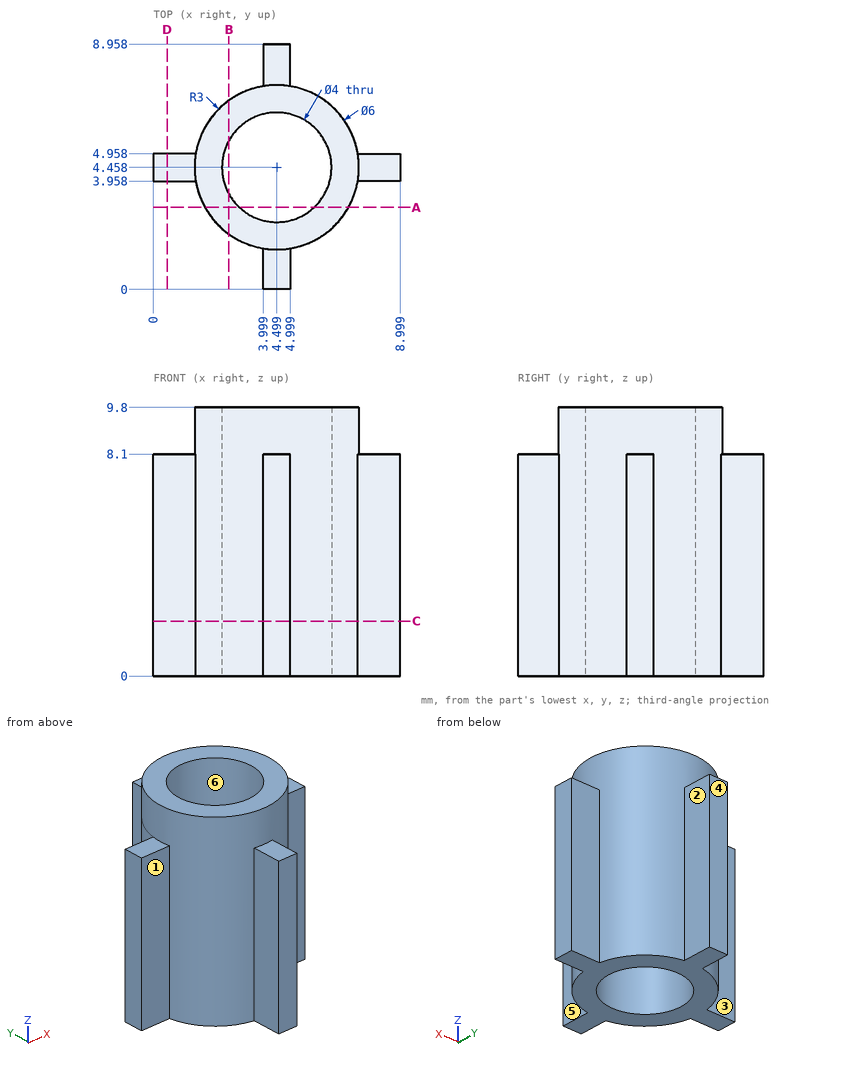
Can you work these out from the drawing? Everything is in mm from the part's minimum corner. A direction names the side the tool comes from. Give positions to 0.01 mm unless a question says otherwise; leave off trailing zeros. Write each loop counter-clockwise with the first axis right and the second up, starting at its lowest first coordinate (ties: lowest second). Pieces come first, ordered by that corner, then holes. Notation, with made-up numbers: (-3, -39.75) -> (24, -39.75) arc R12 ccw to (24, -16.75) -> close; hole circle Ø9 at (52.5, -4). An arc over 180 degrees is marked (long way). Write each question's results on one line, items separated by ' | '. Start each with the question number.
Q1. We'd pull the mould along Y, two halves only. Please class the marked faces 4, 5 and 6: +Y half, -Y half, draft (parallel to the pull), parting line (faces both ways), or undercut.
Q2. Suppose I cut it at A-A, the plane y = 3. List the corners of the cut face in (x, z) for me.
Q3. I'm going to push flat-ended pins straight in: pin 1 Ø0.5 at (x, z) = (8, 4) entering from -Y; pin 2 Ø0.8 at (y, z) = (0.5, 6) entering from +X; pin 3 Ø0.8 at (x, z) = (8.5, 5) entering from +Y. Where does each tip first touch, or does it pass through?
Q4. Suppose I cut it at B-B, the plane x = 2.75. List the corners of the cut face in (y, z) for me.
Q5. I need wall thicknesses on probe 1 along Y at (x, z) = (4.5, 9); probe 2 along X at (y, z) = (4.5, 7); probe 3 along X at (y, z) = (3.5, 9.75) (1 decimal). Which ranges of each line are inside material? Lowest first, please.
Q6. Which directions (+Z, -Z, +X, -X, +Y, -Y) give clear straight access to the entire face, cutting with the end or side of a thin tool? Please do the marked faces 1, 2 and 3.
Q7. Suppose I cut it at D-D, the plane x = 0.5. List the corners of the cut face in (y, z) for me.
Q8. Suppose I cut it at C-C, the plane z = 2. List the corners of the cut face in (x, y) for me, and give its area (3 significant figures).
Outcome:
1) face 4: +Y half | face 5: draft | face 6: undercut
2) outline: (1.88, 0) -> (3.13, 0) -> (3.13, 9.8) -> (1.88, 9.8) -> close; (5.87, 0) -> (7.12, 0) -> (7.12, 9.8) -> (5.87, 9.8) -> close
3) pin 1: y = 3.96 | pin 2: x = 5 | pin 3: y = 4.96
4) outline: (2.02, 0) -> (3.49, 0) -> (3.49, 9.8) -> (2.02, 9.8) -> close; (5.43, 0) -> (6.9, 0) -> (6.9, 9.8) -> (5.43, 9.8) -> close
5) probe 1: 1.46 to 2.46, 6.46 to 7.46 | probe 2: 0 to 2.5, 6.5 to 9 | probe 3: 1.7 to 2.7, 6.3 to 7.3
6) face 1: +Z, -Z, -X, -Y | face 2: +Z, -Z, +X, +Y | face 3: +Z, -Z, -X, +Y
7) outline: (3.96, 0) -> (4.96, 0) -> (4.96, 8.1) -> (3.96, 8.1) -> close
8) outline: (0, 3.96) -> (1.54, 3.96) arc R3 ccw to (4, 1.5) -> (4, 0) -> (5, 0) -> (5, 1.5) arc R3 ccw to (7.46, 3.96) -> (9, 3.96) -> (9, 4.96) -> (7.46, 4.96) arc R3 ccw to (5, 7.42) -> (5, 8.96) -> (4, 8.96) -> (4, 7.42) arc R3 ccw to (1.54, 4.96) -> (0, 4.96) -> close; hole circle Ø4 at (4.5, 4.46) | area: 21.7 mm2
